from build123d import *

# Parameters (mm, degrees)
SKETCH_1_W          = 130
SKETCH_1_H          = 60
EXTRUDE_1_DEPTH     = 3
SKETCH_2_R          = 1.5
CUT_EXTRUDE_1_DEPTH = 3


with BuildPart() as part:
    # Эскиз1 → Бобышка-Вытянуть1 (new body)
    with BuildSketch(Plane(origin=(0, 0, 0), x_dir=(1, 0, 0), z_dir=(0, 1, 0))):
        Rectangle(SKETCH_1_W, SKETCH_1_H)
    extrude(amount=EXTRUDE_1_DEPTH)

    # Эскиз2 → Вырез-Вытянуть1 (cut)
    with BuildSketch(Plane(origin=(0, 3, 0), x_dir=(1, 0, 0), z_dir=(0, 1, 0))):
        with Locations((-56.052735869, 17)):
            Circle(SKETCH_2_R)
        with Locations((-40.052735869, 17)):
            Circle(SKETCH_2_R)
        with Locations((-24.052735869, 17)):
            Circle(SKETCH_2_R)
        with Locations((-8.052735869, 17)):
            Circle(SKETCH_2_R)
        with Locations((7.947264131, 17)):
            Circle(SKETCH_2_R)
        with Locations((23.947264131, 17)):
            Circle(SKETCH_2_R)
        with Locations((39.947264131, 17)):
            Circle(SKETCH_2_R)
        with Locations((55.947264131, 17)):
            Circle(SKETCH_2_R)
        with Locations((-56.052735869, 0)):
            Circle(SKETCH_2_R)
        with Locations((-56.052735869, -17)):
            Circle(SKETCH_2_R)
        with Locations((-40.052735869, 0)):
            Circle(SKETCH_2_R)
        with Locations((-40.052735869, -17)):
            Circle(SKETCH_2_R)
        with Locations((-24.052735869, 0)):
            Circle(SKETCH_2_R)
        with Locations((-24.052735869, -17)):
            Circle(SKETCH_2_R)
        with Locations((-8.052735869, 0)):
            Circle(SKETCH_2_R)
        with Locations((-8.052735869, -17)):
            Circle(SKETCH_2_R)
        with Locations((7.947264131, 0)):
            Circle(SKETCH_2_R)
        with Locations((7.947264131, -17)):
            Circle(SKETCH_2_R)
        with Locations((23.947264131, 0)):
            Circle(SKETCH_2_R)
        with Locations((23.947264131, -17)):
            Circle(SKETCH_2_R)
        with Locations((39.947264131, 0)):
            Circle(SKETCH_2_R)
        with Locations((39.947264131, -17)):
            Circle(SKETCH_2_R)
        with Locations((55.947264131, 0)):
            Circle(SKETCH_2_R)
        with Locations((55.947264131, -17)):
            Circle(SKETCH_2_R)
    extrude(amount=-CUT_EXTRUDE_1_DEPTH, mode=Mode.SUBTRACT)


solid = part.part
Here's how the part is built. I have some questions about the finished solid (model axes, mm). Give positions to 0.01 mm unless a question says otherwise; leave off trailing zeros. One line per item, written item: value. Start each with the question number.
1. Imagine slicing it at A-A, the plane y = 1.35. Count the separate pieces of the cut face and the enclosed holes in it, plus the area to 3 significant figures.
2. I need wall thicknesses on probe 1 along Z at (x, y) = (7.5, 1.5). Which ranges of the line are inside material? Lowest first, please. Write a range as from..to.
3. We'd pull the mould along X, two halves only. Please class faces 1 (the face through (65, 1, 0)), 2 (the face through (-7.246, 1.521, 15.735)), 3 (the face through (-1, 0, 0)): released by +X, released by -X, zero draft, split by the parting line, or undercut.
Values follow:
1. separate pieces: 1
1. enclosed holes: 24
1. area: 7,630 mm2
2. probe 1: z = -30..-18.43, -15.57..-1.43, 1.43..15.57, 18.43..30
3. face 1: released by +X
3. face 2: undercut
3. face 3: zero draft
